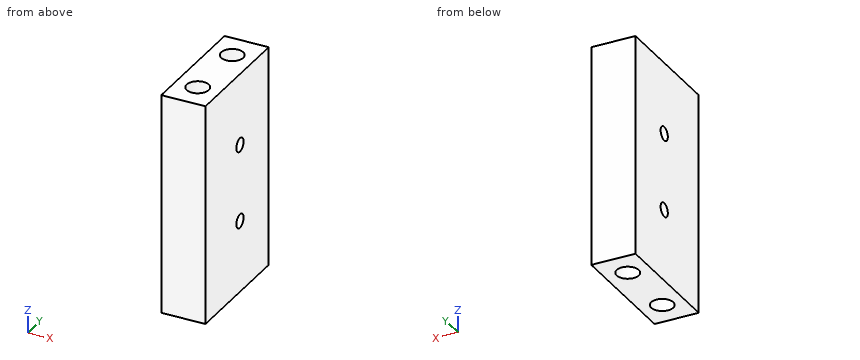
from build123d import *

# Parameters (mm, degrees)
SKETCH1_W           = 127
SKETCH1_H           = 69.85
BOSS_EXTRUDE1_DEPTH = 25.4
SKETCH2_R           = 6.35
CUT_EXTRUDE1_DEPTH  = 25.4
SKETCH3_R           = 3.96875
CUT_EXTRUDE2_DEPTH  = 26.4


with BuildPart() as part:
    # Sketch1 → Boss-Extrude1 (new body)
    with BuildSketch(Plane(origin=(0, 0, 0), x_dir=(0, 0, -1), z_dir=(1, 0, 0))):
        Rectangle(SKETCH1_W, SKETCH1_H)
    extrude(amount=BOSS_EXTRUDE1_DEPTH)

    # Sketch2 → Cut-Extrude1 (cut)
    with BuildSketch(Plane.XY.offset(63.5)):
        with Locations((12.7, 19.05)):
            Circle(SKETCH2_R)
        with Locations((12.7, -19.05)):
            Circle(SKETCH2_R)
    cut_extrude1 = extrude(amount=-CUT_EXTRUDE1_DEPTH, mode=Mode.SUBTRACT)

    # Mirror1: Cut-Extrude1 across plane
    add(cut_extrude1.mirror(Plane.XY), mode=Mode.SUBTRACT)

    # Sketch3 → Cut-Extrude2 (cut, through all)
    with BuildSketch(Plane(origin=(25.4, 0, 0), x_dir=(0, 0, -1), z_dir=(1, 0, 0))):
        with Locations((-22.225, 3.175)):
            Circle(SKETCH3_R)
        with Locations((22.225, 3.175)):
            Circle(SKETCH3_R)
    extrude(amount=-CUT_EXTRUDE2_DEPTH, mode=Mode.SUBTRACT)


solid = part.part
Part model, mm, in its own coordinate system. Give positions to 0.01 mm unless a question says otherwise; leave off trailing zeros. Order: outer loops, then holes, each group sorted by start corner. A loop starts at its lowest first (then second) coordinate and runs counter-clockwise, first axis right, second up. Notation, with made-up numbers: (5, 11.25) -> (52, 11.25) arc R22 cw to (52, 23.25) -> close; hole circle Ø1 at (5.25, 32). An arc over 180 degrees is marked (long way). Use one line per item in the form item = value.
(1) Flat gauge pins, fed straight in: P1, Ø8, axis at y = -15, z = -12.5, coming from the -X side; P2, Ø11.5, axis at x = 12.7, y = 19.05, coming from the -Z side; P3, Ø4, axis at x = 12.5, y = -21.5, coming from the +Z side. Where does each tip first touch, or does it go through?
Solution:
P1 = 0
P2 = -38.1
P3 = 38.1
(2) Drill centre lines: line 1 (Y direction, x = 12.7, z = -47) (3 decimals); line 2 (Y direction, x = 16.5, z = 49) (3 decimals); line 3 (X direction, y = 19, z = -50). Where is each one in solid material? Low to high. Write a range as from..to.
Solution:
line_1 = -34.925..-25.4, -12.7..12.7, 25.4..34.925
line_2 = -34.925..-24.137, -13.963..13.963, 24.137..34.925
line_3 = 0..6.35, 19.05..25.4
(3) Saw through at A-A (z = 55.5). Write the cut outline in (x, y) (3 decimals), then the cut area to 3 significant figures.
Solution:
outline = (0, -34.925) -> (25.4, -34.925) -> (25.4, 34.925) -> (0, 34.925) -> close; hole circle Ø12.7 at (12.7, -19.05); hole circle Ø12.7 at (12.7, 19.05)
area = 1,520 mm²
(4) Saw through at B-B (z = -23.5). Write the cut outline in (x, y) (3 decimals).
Solution:
outline = (0, -34.925) -> (25.4, -34.925) -> (25.4, -0.583) -> (0, -0.583) -> close; (0, 6.933) -> (25.4, 6.933) -> (25.4, 34.925) -> (0, 34.925) -> close
(5) Saw through at C-C (y = -17). Write the cut outline in (x, z).
Solution:
outline = (0, -63.5) -> (6.69, -63.5) -> (6.69, -38.1) -> (18.71, -38.1) -> (18.71, -63.5) -> (25.4, -63.5) -> (25.4, 63.5) -> (18.71, 63.5) -> (18.71, 38.1) -> (6.69, 38.1) -> (6.69, 63.5) -> (0, 63.5) -> close
